The listing builds one solid part. Answer for the finished solid, in the listing's coordinates (mm). A direction names the side the tool comes from. Coordinates: 2 decimals unless noted, no trailing zeros. Order: outer loops, then holes, each group sorted by start corner. A loop starts at its lowest first (then second) coordinate and runs counter-clockwise, first axis right, second up. Notation, with made-up numbers: (25.25, 49.5) - (53.25, 49.5) arc R21 cw to (53.25, 82.5) - close; hole circle Ø2 at (74, -8). An arc over 180 degrees is marked (long way). Use one line per item in the form item = value. Start each with the question number.
Item 1: Section B-B, the plane x = 35 is taken. Write down the section's boundary in (y, z).
Item 2: A tool of negligible diameter and unlimited length cuts with its end or side. For faces 4 (the cylindrical face through (-52.69, -3.99, 54.04)), 5 (the flat face through (-60, -1, -1)), from which of +Z, -Z, +X, -X, +Y, -Y can it reach the whole face along a straight path? Write none if from no direction.
Item 3: Section A-A, the plane z = -55 is taken. Write down the section's boundary in (x, y).
Item 4: The mould has two halves that part along Z. Classify faces 1 (the flat face through (-1, -1.1, 1)), 2 (the flat face through (-1, -1, 60)), 3 (the flat face through (-1, 0, 1)): released by +Z, released by -Z, zero draft, split by the parting line, or undercut.
Item 5: This flat-tipped pin is pushed along its axis until it touches: pin 1 Ø2 at (x, z) = (3.5, 36.5) entering from -Y. Where does it stop, or does it pass through?
Item 6: Consider line 1 along Z through (x, y) = (31.5, -2.9); line 2 along Y through (x, z) = (54, -49). Determine where each line is inside the solid, lowest interval first. Write a range as [from, to].
from build123d import *

# Parameters (mm, degrees)
F0_W     = 120
F0_H     = 120
F0_W_2   = 102
F0_H_2   = 102
F1_DEPTH = 3
F2_DEPTH = 1.1
F3_R     = 2.5
F4_DEPTH = 2


with BuildPart() as f1:
    # F0 (on Front) → F1 (new body)
    with BuildSketch(Plane.XZ):
        Rectangle(F0_W, F0_H)
        Rectangle(F0_W_2, F0_H_2, mode=Mode.SUBTRACT)
    extrude(amount=F1_DEPTH)

    # F0 (on Front) → F2 (join)
    with BuildSketch(Plane.XZ):
        Rectangle(F0_W_2, F0_H_2)
    extrude(amount=F2_DEPTH)

    # F3 (on face) → F4 (join)
    with BuildSketch(Plane.XZ.offset(3)):
        with Locations((-55, 55)):
            Circle(F3_R)
        with Locations((55, -55)):
            Circle(F3_R)
    extrude(amount=F4_DEPTH)


solid = f1.part
Response:
q1.outline = (-3, -60) - (0, -60) - (0, 60) - (-3, 60) - (-3, 51) - (-1.1, 51) - (-1.1, -51) - (-3, -51) - close
q2.face_4 = -Y
q2.face_5 = +Z, -Z, -X, +Y, -Y
q3.outline = (-60, -3) - (52.5, -3) - (52.5, -5) - (57.5, -5) - (57.5, -3) - (60, -3) - (60, 0) - (-60, 0) - close
q4.face_1 = undercut
q4.face_2 = released by +Z
q4.face_3 = zero draft
q5.pin_1 = -1.1
q6.line_1 = [-60, -51], [51, 60]
q6.line_2 = [-3, 0]
